The figure shows three views and two pictorial views of one solid part (mm, origin at its lowest corner). Answer the questions. A direction names the side the tool comes from. Round coordinates to 2 decimals unless told otherwise and drop trailing zeros. Order: outer loops, then holes, each group sorted by start corner. A loop starts at its lowest first (then second) coordinate and runs counter-clockwise, first axis right, second up. Notation, with made-up numbers: (79.25, 65) -> (90.25, 65) arc R21 ccw to (90.25, 76) -> close; hole circle Ø3 at (-1, 3.25). An arc over 180 degrees is marked (long way). Return JSON: item names as keys, results as strings. Group by question number.
(1) The part is cut by section D-D (y = 26). Determine the outline of the cut face in (x, z).
(2) The part is cut by section C-C (x = 3). Determine the outline of the cut face in (y, z).
(3) Each of these flat-tipped pins is pushed along its axis until it touches: pin 1 (4 mm diameter, centred on x = 14, y = 12, fed in from +Z); pin 2 (4 mm diameter, centred on x = 16, y = 20, fed in from -Z); pin 3 (1 mm diameter, centred on x = 16, z = 13.5, fed in from -Y); pin 4 (3 mm diameter, centred on x = 3, y = 7, fed in from +Z). Where does it stop, or does it pass through?
(4) Consider line 1 (Y direction, x = 3, z = 24); line 2 (X direction, y = 3, z = 34.5); line 3 (X direction, y = 23.5, z = 14). Determine where each line is inside the solid, lowest interval first. Write a range as [from, to].
(5) The part is cut by section B-B (z = 20.5). Determine the outline of the cut face in (x, y), plus the area to 3 significant figures.
(6) The part is cut by section A-A (y = 7). Determine the outline of the cut face in (x, z).
(7) Which of the six approach directions +Z, -Z, +X, -X, +Y, -Y give full straight-line access (tool end or side, diameter ignored) to the marked faces 4, 5, 6, 7 and 8?
(8) Determine the mould class of the marked faces 1, 2 and 3 for opening direction X: +X half, -X half, draft (parallel to the pull), parting line (faces both ways), or undercut.
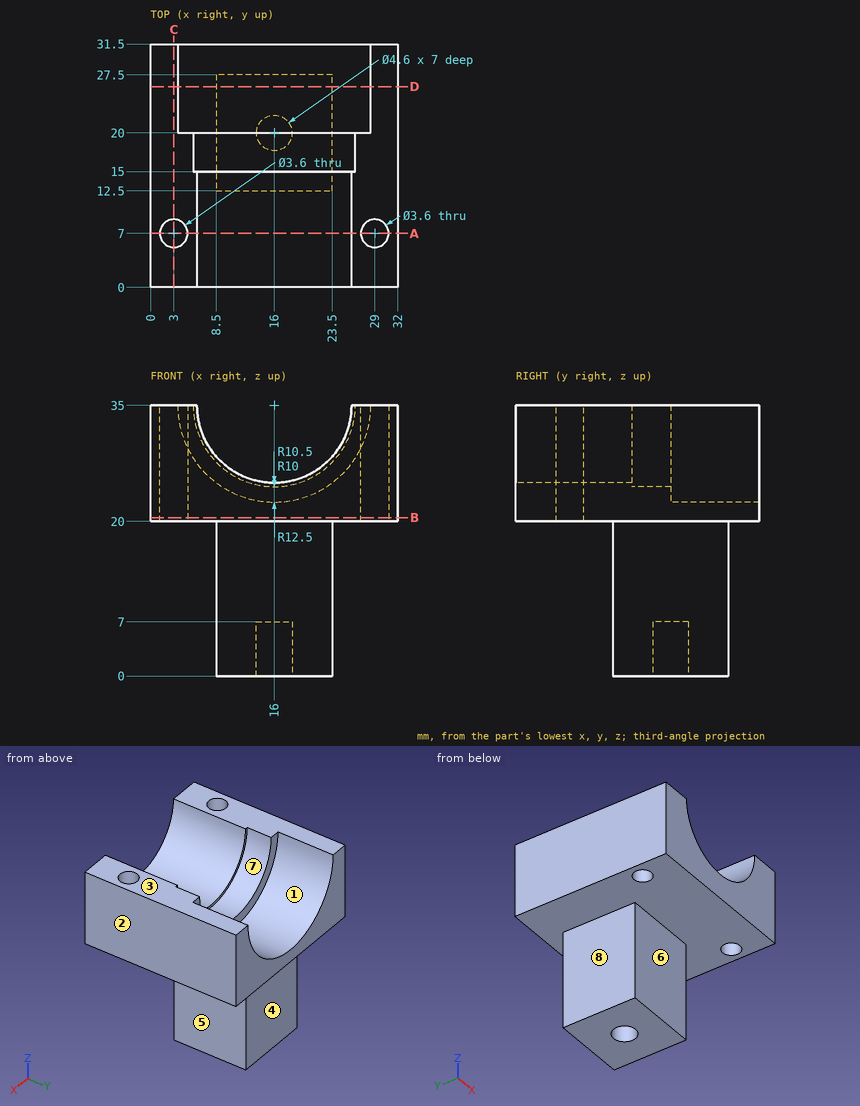
Answer below:
{
 "1": {"outline": "(0, 20) -> (8.5, 20) -> (8.5, 0) -> (23.5, 0) -> (23.5, 20) -> (32, 20) -> (32, 35) -> (28.5, 35) arc R12.5 cw to (3.5, 35) -> (0, 35) -> close"},
 "2": {"outline": "(0, 20) -> (5.2, 20) -> (5.2, 35) -> (0, 35) -> close; (8.8, 20) -> (31.5, 20) -> (31.5, 35) -> (8.8, 35) -> close"},
 "3": {"pin 1": "stops at z = 25.83", "pin 2": "stops at z = 7", "pin 3": "stops at y = 12.5", "pin 4": "passes through"},
 "4": {"line 1": "y = [0, 5.2], [8.8, 31.5]", "line 2": "x = [0, 6.01], [25.99, 32]", "line 3": "x = [8.5, 23.5]"},
 "5": {"outline": "(0, 0) -> (32, 0) -> (32, 31.5) -> (0, 31.5) -> close; hole circle Ø3.6 at (3, 7); hole circle Ø3.6 at (29, 7)", "area": "988 mm²"},
 "6": {"outline": "(0, 20) -> (1.2, 20) -> (1.2, 35) -> (0, 35) -> close; (4.8, 20) -> (27.2, 20) -> (27.2, 35) -> (26, 35) arc R10 cw to (6, 35) -> (4.8, 35) -> close; (30.8, 20) -> (32, 20) -> (32, 35) -> (30.8, 35) -> close"},
 "7": {"face 4": "-Z, +X, -X, +Y", "face 5": "-Z, +X, +Y, -Y", "face 6": "-Z, +X, -X, -Y", "face 7": "+Z, +Y", "face 8": "-Z, -X, +Y, -Y"},
 "8": {"face 1": "undercut", "face 2": "+X half", "face 3": "draft"}
}
